```python
from build123d import *

# Parameters (mm, degrees)
SKETCH1_W                        = 508
SKETCH1_H                        = 508
BOSS_EXTRUDE1_DEPTH              = 12.7
K_0_281_DIAMETER_HOLE1_D         = 7.1374
K_0_281_DIAMETER_HOLE1_DEPTH     = 12.7
F_5_8_0_625_DIAMETER_HOLE1_D     = 15.875
F_5_8_0_625_DIAMETER_HOLE1_DEPTH = 25.4
F_5_8_0_625_DIAMETER_HOLE1_TIP   = 4.769331164


with BuildPart() as part:
    # Sketch1 → Boss-Extrude1 (new body)
    with BuildSketch(Plane(origin=(0, 0, 0), x_dir=(1, 0, 0), z_dir=(0, 1, 0))):
        Rectangle(SKETCH1_W, SKETCH1_H)
    extrude(amount=BOSS_EXTRUDE1_DEPTH)

    # K (0.281) Diameter Hole1
    with Locations(Plane(origin=(0, 12.7, 0), x_dir=(1, 0, 0), z_dir=(0, 1, 0))):
        with Locations((-77.47, -228.6), (-77.47, -172.72), (77.47, -172.72), (77.47, -228.6), (-228.6, -77.47), (-172.72, -77.47), (-172.72, 77.47), (-228.6, 77.47)):
            Hole(K_0_281_DIAMETER_HOLE1_D / 2, depth=K_0_281_DIAMETER_HOLE1_DEPTH)

    # 5/8 (0.625) Diameter Hole1
    with Locations(Plane(origin=(0, 12.7, 0), x_dir=(1, 0, 0), z_dir=(0, 1, 0))):
        with Locations((0, 0)):
            Hole(F_5_8_0_625_DIAMETER_HOLE1_D / 2, depth=F_5_8_0_625_DIAMETER_HOLE1_DEPTH)
            with Locations((0, 0, -(F_5_8_0_625_DIAMETER_HOLE1_DEPTH + F_5_8_0_625_DIAMETER_HOLE1_TIP / 2))):  # 118° drill point
                Cone(0, F_5_8_0_625_DIAMETER_HOLE1_D / 2, F_5_8_0_625_DIAMETER_HOLE1_TIP, mode=Mode.SUBTRACT)


solid = part.part
```
Could you check a few things on this model? Use its own coordinates, in mm. Give positions to 0.01 mm unless a question says otherwise; leave off trailing zeros. Loops run counter-clockwise (first coordinate to the right, second up) from the corner with the lowest first, then second, coordinate; pieces in that order, holes last. Notation, with made-up numbers: (86.5, 78.5) -> (107.5, 78.5) arc R15 cw to (107.5, 91.5) -> close; hole circle Ø3 at (0.5, -3.75). An arc over 180 degrees is marked (long way). Put each result on its own line as item: value.
(1) Please list where these lines run through material, in increasing order: probe 1 along Z at (x, y) = (-77.47, 4); probe 2 along X at (y, z) = (5.75, -77.47); probe 3 along Z at (x, y) = (-172.72, 9.5). Write a range as [from, to].
Computed:
probe 1: [-254, 169.15], [176.29, 225.03], [232.17, 254]
probe 2: [-254, -232.17], [-225.03, -176.29], [-169.15, 254]
probe 3: [-254, -81.04], [-73.9, 73.9], [81.04, 254]
(2) Thinking about a two-plate mould opening in X: for faces 1 (the face through (1.72, 6.26, 7.75)), 2 (the face through (-4, 6, 254)), 3 (the face through (-254, 6, 4)), which applies, pulls with the +X half, pulls with the -X half, needs draft (parallel to the pull), parting line crosses it, or undercut?
Computed:
face 1: undercut
face 2: needs draft
face 3: pulls with the -X half
(3) I'm going to push flat-ended pins straight in: pin 1 Ø4.5 at (x, z) = (-172.72, 77.47) entering from -Y; pin 2 Ø11.5 at (x, z) = (-77.47, 172.72) entering from +Y. Where does each tip first touch, or does it pass through?
Computed:
pin 1: through
pin 2: y = 12.7
(4) Imagine slicing it at B-B on z = 0. Write out the boundary of the cut face in (x, y), plus the area to 3 significant figures.
Computed:
outline: (-254, 0) -> (-7.94, 0) -> (-7.94, 12.7) -> (-254, 12.7) -> close; (7.94, 0) -> (254, 0) -> (254, 12.7) -> (7.94, 12.7) -> close
area: 6,250 mm^2
(5) Imagine slicing it at A-A on x = 0. Write out the boundary of the cut face in (y, z).
Computed:
outline: (0, -254) -> (12.7, -254) -> (12.7, -7.94) -> (0, -7.94) -> close; (0, 7.94) -> (12.7, 7.94) -> (12.7, 254) -> (0, 254) -> close
